CAD build for the part. Positions are in the model's coordinates, mm. A direction names the side the tool comes from. Coordinates: 2 decimals unless noted, no trailing zeros. Write each loop counter-clockwise with the first axis right and the second up, starting at its lowest first coordinate (ties: lowest second). Pieces come first, ordered by that corner, then holes. Notation, with made-up numbers: (24.5, -12) - (62.5, -12) arc R23 ccw to (62.5, 22) - close; hole circle Ø8 at (-12.5, 27). An arc over 180 degrees is marked (long way). Answer in a Markdown table with one row per item. Add a question column.
Q1. Pin check, flat tips, straight feed: pin 1 (4 mm diameter, centred on y = 20.5, z = 8, fed in from -X); pin 2 (4 mm diameter, centred on y = 20, z = 14, fed in from +X); pin 3 (12 mm diameter, centred on x = 19.5, z = 39, fed in from +Y); pin 4 (1 mm diameter, centred on y = 18, z = 13.5, fed in from +X). Stop position of each tip, or through.
Q2. Two-plate mould, pull along Z, no slides. Class faces 3 (the flat face through (3, 21, -2.795)), 4 (the flat face through (-40.358, 10, 30)), 5 (the flat face through (3, 21, 31.833)): +Z half, -Z half, draft (parallel to the pull), parting line (faces both ways), or undercut.
Q3. Drill centre lines: line 1 along Y through (x, z) = (-32, 17.5); line 2 along Y through (x, z) = (48.5, 49); line 3 along Y through (x, z) = (13.5, 2). Where is each one in solid material? Low to high. Write a range as from..to.
Q4. Band-saw the part on C-C (y = 16). List the corners of the cut face in (x, z), and give its area (3 significant figures).
Q5. 3-axis set-ups, long thin cutter, end or side, ignore diameter. For faces 1 (the flat face through (-40.575, 21, 14)), 2 (the flat face through (2, -2, 7.739)): which of +Z, -Z, +X, -X, +Y, -Y reach the whole face in a straight line?
Q6. Band-saw the part on A-A (z = 15.5). List the corners of the cut face in (x, y).
Q7. Band-saw the part on D-D (z = 2). List the corners of the cut face in (x, y), and give its area (3 significant figures).
```python
from build123d import *

# Parameters (mm, degrees)
F0_W     = 152.4
F0_H     = 63.5
F1_DEPTH = 3.81
F3_W     = 88.9
F3_H     = 19.812
F4_DEPTH = 3.81
F6_W     = 89.090503
F6_H     = 34.628688
F7_DEPTH = 3.81


with BuildPart() as f1:
    # F0 (on Front) → F1 (new body)
    with BuildSketch(Plane.XZ):
        with Locations((3.185697, 39.488637)):
            Rectangle(F0_W, F0_H)
    extrude(amount=F1_DEPTH)

    # F3 (on offset) → F4 (join)
    with BuildSketch(Plane.XY.offset(28.0416)):
        with Locations((4.091607, 9.906)):
            Rectangle(F3_W, F3_H)
    extrude(amount=F4_DEPTH)

    # F6 (on offset) → F7 (join)
    with BuildSketch(Plane.XZ.offset(-22.86)):
        with Locations((3.969803, 14.518858)):
            Rectangle(F6_W, F6_H)
    extrude(amount=F7_DEPTH)


solid = f1.part
```
Checked values:
| question | item | result |
|---|---|---|
| 1 | pin 1 | stops at x = -40.58 |
| 1 | pin 2 | stops at x = 48.52 |
| 1 | pin 3 | stops at y = 0 |
| 1 | pin 4 | passes through |
| 2 | face 3 | -Z half |
| 2 | face 4 | draft |
| 2 | face 5 | +Z half |
| 3 | line 1 | y = -3.81..0, 19.05..22.86 |
| 3 | line 2 | y = -3.81..0 |
| 3 | line 3 | y = 19.05..22.86 |
| 4 | outline | (-40.36, 28.04) - (48.54, 28.04) - (48.54, 31.85) - (-40.36, 31.85) - close |
| 4 | area | 339 mm² |
| 5 | face 1 | +Z, -Z, -X, +Y |
| 5 | face 2 | -Z, +X, -X, -Y |
| 6 | outline | (-73.01, -3.81) - (79.39, -3.81) - (79.39, 0) - (-73.01, 0) - close; (-40.58, 19.05) - (48.52, 19.05) - (48.52, 22.86) - (-40.58, 22.86) - close |
| 7 | outline | (-40.58, 19.05) - (48.52, 19.05) - (48.52, 22.86) - (-40.58, 22.86) - close |
| 7 | area | 339 mm² |
